Verification items for the finished model (mm, model axes). A direction names the side the tool comes from. Give positions to 0.01 mm unless a question says otherwise; leave off trailing zeros. Write each loop counter-clockwise with the first axis right and the second up, starting at its lowest first coordinate (ties: lowest second). Pieces come first, ordered by that corner, then holes. Notation, with made-up numbers: (87, 0) -> (109, 0) arc R21 ccw to (109, 17) -> close; hole circle Ø7 at (76.25, -35.75). An arc over 180 degrees is marked (long way). Answer as CSV lines item,"result". Start each with the question number.
1) Sectioned sample at B-B on x = 0. Record the cut outline in (y, z), and give its area (3 significant figures).
2) Gauge pin test, flat ends, axial feed: pin 1 Ø3 at (x, z) = (27, 1492) entering from +Y; pin 2 Ø12 at (x, y) = (1, -26.5) entering from -Z; pin 3 Ø8 at (y, z) = (5.5, 1199) entering from -X. Record the tip position at first contact, or that the pin passes through.
3) Sectioned sample at C-C on z = 617.5. Record the cut outline in (x, y), and give its area (3 significant figures).
4) Tool access check on faces 5 (the flat face through (1, 15, -23)), 6 (the flat face through (1, -15, -23)), 7 (the flat face through (0, 0, 30)). Record the directions out of +Z, -Z, +X, -X, +Y, -Y that give a thin tool (end or side, any length) a straight path to the whole face; none if there is none.
5) Mould release check, pull along X, two halves, no side actions. Record for faces 1 (the cylindrical face through (-4.336, -19.524, 1001.21)), 2 (the cylindrical face through (47.69, 15.02, 986)), 3 (the cylindrical face through (-10.648, -0.21, -58.887)), 4 (the flat face through (-1, -22, 2000)): released by +X, released by -X, zero draft, split by the parting line, or undercut.
6) Material ranges on L1, parallel to X at y = 0.5, z = 280.5; L2, parallel to Y at x = 0, z = 763; L3, parallel to Z at x = -15.5, y = 46.5, recorded low to high.
7) Sectioned sample at A-A on y = 0. Record the cut outline in (x, z), and give its area (3 significant figures).
```python
from build123d import *

# Parameters (mm, degrees)
SKETCH1_R           = 50
BOSS_EXTRUDE1_DEPTH = 2000
SHELL1_T            = -30
SKETCH2_R           = 17.5
BOSS_EXTRUDE2_DEPTH = 15


with BuildPart() as part:
    # Sketch1 → Boss-Extrude1 (new body)
    with BuildSketch(Plane.XY):
        Circle(SKETCH1_R)
    extrude(amount=BOSS_EXTRUDE1_DEPTH)

    # Shell1
    shell1_openings = [part.faces().sort_by_distance(p)[0] for p in [
        (0, 0, 2000),
    ]]
    offset(amount=SHELL1_T, openings=shell1_openings, kind=Kind.INTERSECTION)

    # Sketch2 → Boss-Extrude2 (add, symmetric)
    with BuildSketch(Plane(origin=(0, 0, 0), x_dir=(1, 0, 0), z_dir=(0, 1, 0))):
        with BuildLine():
            Line((-45, 0), (-34.28083908, 52.058616858))
            ThreePointArc((-34.28083908, 52.058616858), (0, 80), (34.28083908, 52.058616858))
            Line((34.28083908, 52.058616858), (45, 0))
            Line((45, 0), (-45, 0))
        make_face()
        with Locations(Location((0, 45, 0), (0, 0, 270))):
            Circle(SKETCH2_R, mode=Mode.SUBTRACT)
    extrude(amount=BOSS_EXTRUDE2_DEPTH, both=True)


solid = part.part
```
Ans:
1,outline,"(-50, 0) -> (-15, 0) -> (-15, -27.5) -> (15, -27.5) -> (15, 0) -> (50, 0) -> (50, 2000) -> (20, 2000) -> (20, 30) -> (-20, 30) -> (-20, 2000) -> (-50, 2000) -> close; (-15, -80) -> (15, -80) -> (15, -62.5) -> (-15, -62.5) -> close"
1,area,"123,000 mm²"
2,pin 1,"stops at y = 43.01"
2,pin 2,"stops at z = 0"
2,pin 3,"stops at x = -49.98"
3,outline,"circle Ø100 at (0, 0); hole circle Ø40 at (0, 0)"
3,area,"6,600 mm²"
4,face 5,"-Z, +X, -X, +Y"
4,face 6,"-Z, +X, -X, -Y"
4,face 7,"+Z"
5,face 1,"undercut"
5,face 2,"split by the parting line"
5,face 3,"undercut"
5,face 4,"zero draft"
6,L1,"x = -50 to -19.99, 19.99 to 50"
6,L2,"y = -50 to -20, 20 to 50"
6,L3,"z = 0 to 2000"
7,outline,"(-50, 0) -> (-45, 0) -> (-34.28, -52.06) arc R35 ccw to (34.28, -52.06) -> (45, 0) -> (50, 0) -> (50, 2000) -> (20, 2000) -> (20, 30) -> (-20, 30) -> (-20, 2000) -> (-50, 2000) -> close; hole circle Ø35 at (0, -45)"
7,area,"126,000 mm²"
